```python
from build123d import *

# Parameters (mm, degrees)
F0_R     = 6.35
F1_DEPTH = 6.35


with BuildPart() as f1:
    # F0 (on Front) → F1 (new body)
    with BuildSketch(Plane.XZ):
        with BuildLine():
            ThreePointArc((81.650485, 2.54), (78.67469, 9.724205), (71.490485, 12.7))
            Line((71.490485, 12.7), (-91.44, 12.7))
            ThreePointArc((-91.44, 12.7), (-98.624205, 9.724205), (-101.6, 2.54))
            Line((-101.6, 2.54), (-101.6, -2.54))
            ThreePointArc((-101.6, -2.54), (-98.624205, -9.724205), (-91.44, -12.7))
            Line((-91.44, -12.7), (71.490485, -12.7))
            ThreePointArc((71.490485, -12.7), (78.67469, -9.724205), (81.650485, -2.54))
            Line((81.650485, -2.54), (81.650485, 2.54))
        make_face()
        with Locations((-91.44, 0)):
            Circle(F0_R, mode=Mode.SUBTRACT)
        Circle(F0_R, mode=Mode.SUBTRACT)
        with Locations((66.04, 0)):
            Circle(F0_R, mode=Mode.SUBTRACT)
    extrude(amount=F1_DEPTH)


solid = f1.part
```
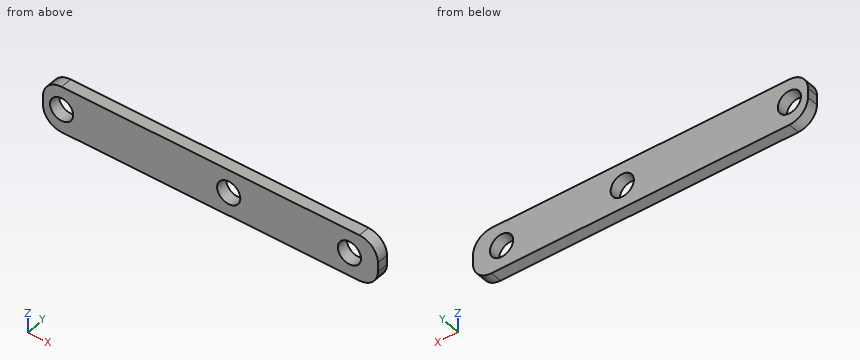
Model file for the job. Use its own axes, mm. Give positions to 0.01 mm unless a question says otherwise; leave off trailing zeros. Write each loop counter-clockwise with the first axis right and the second up, starting at its lowest first coordinate (ties: lowest second). Pieces come first, ordered by that corner, then holes. Notation, with made-up numbers: M -37,24 L -1,24 A22 cw -1,39 Z; hole C -25,-6.75 d8. An arc over 180 degrees is marked long. Use a Markdown table: item, result.
1) Drill centre lines: line 1 (Z direction, x = -91.44, y = -2.5); line 2 (X direction, y = -1.75, z = -0.75); line 3 (X direction, y = -1.5, z = 1.5). Where is each one in solid material? Low to high. Write a range as from..to.
Responses:
| item | result |
|---|---|
| line 1 | z = -12.7..-6.35, 6.35..12.7 |
| line 2 | x = -101.6..-97.75, -85.13..-6.31, 6.31..59.73, 72.35..81.65 |
| line 3 | x = -101.6..-97.61, -85.27..-6.17, 6.17..59.87, 72.21..81.65 |
2) Cut at A-A (y = -2.75). List the corners of the cut face in (x, z).
Responses:
| item | result |
|---|---|
| outline | M -101.6,-2.54 A10.16 ccw -91.44,-12.7 L 71.49,-12.7 A10.16 ccw 81.65,-2.54 L 81.65,2.54 A10.16 ccw 71.49,12.7 L -91.44,12.7 A10.16 ccw -101.6,2.54 Z; hole C -91.44,0 d12.7; hole C 0,0 d12.7; hole C 66.04,0 d12.7 |
3) Cut at B-B (z = 0). List the corners of the cut face in (x, y).
Responses:
| item | result |
|---|---|
| outline | M -101.6,-6.35 L -97.79,-6.35 L -97.79,0 L -101.6,0 Z; M -85.09,-6.35 L -6.35,-6.35 L -6.35,0 L -85.09,0 Z; M 6.35,-6.35 L 59.69,-6.35 L 59.69,0 L 6.35,0 Z; M 72.39,-6.35 L 81.65,-6.35 L 81.65,0 L 72.39,0 Z |
4) Cut at C-C (x = 66.04). List the corners of the cut face in (y, z), and give its area (3 significant figures).
Responses:
| item | result |
|---|---|
| outline | M -6.35,-12.7 L 0,-12.7 L 0,-6.35 L -6.35,-6.35 Z; M -6.35,6.35 L 0,6.35 L 0,12.7 L -6.35,12.7 Z |
| area | 80.6 mm2 |
5) Pin check, flat tips, straight feed: pin 1 (10 mm diameter, centred on x = -91.44, z = 0, fed in from -Y); pin 2 (1.5 mm diameter, centred on y = -4.5, z = -6, fed in from +X). Stop position of each tip, or through.
Responses:
| item | result |
|---|---|
| pin 1 | passes through |
| pin 2 | stops at x = 81.28 |
6) Cut at D-D (z = 10.5). List the corners of the cut face in (x, y), and give its area (3 significant figures).
Responses:
| item | result |
|---|---|
| outline | M -97.75,-6.35 L 77.8,-6.35 L 77.8,0 L -97.75,0 Z |
| area | 1,110 mm2 |
